```python
from build123d import *

# Parameters (mm, degrees)
SKETCH1_R                   = 12.5
BOSS_EXTRUDE1_DEPTH         = 6.5
CIRPATTERN1_COUNT           = 4
SKETCH5_R                   = 4.5
BOSS_EXTRUDE3_DEPTH         = 6.5
SKETCH7_R                   = 4.1
CUT_EXTRUDE2_DEPTH          = 3
CIRPATTERN3_COUNT           = 2
FILLET2_R                   = 5
M3_TAPPED_HOLE1_D           = 2.5
M3_TAPPED_HOLE1_CSINK_D     = 3.05
M3_TAPPED_HOLE1_CSINK_ANGLE = 90


with BuildPart() as part:
    # Sketch1 → Boss-Extrude1 (new body)
    with BuildSketch(Plane.XY):
        with Locations(Location((0, 0, 0), (0, 0, 180))):
            Circle(SKETCH1_R)
    extrude(amount=BOSS_EXTRUDE1_DEPTH)

    # Sketch4 → CBORE for M3 Hexagon socket head cap screws1 (revolve, cut)
    with BuildSketch(Plane(origin=(-9, 0, 6.5), x_dir=(0, -1, 0), z_dir=(1, 0, 0))):
        Polygon((0, 0), (0, 6.5), (1.6, 6.5), (1.6, 3.4), (3, 3.4), (3, 0.025), (3.025, 0), align=None)
    cbore_for_m3_hexagon_socket_head_cap_scr = revolve(axis=Axis((-9, 0, 12.85), (0, 0, -1)), mode=Mode.SUBTRACT)

    # CirPattern1: CBORE for M3 Hexagon socket head cap screws1 ×4 about axis
    cirpattern1_axis = Axis((0, 0, 0), (0, 0, 1))
    for i in range(1, CIRPATTERN1_COUNT):
        add(cbore_for_m3_hexagon_socket_head_cap_scr.rotate(cirpattern1_axis, i * 360 / CIRPATTERN1_COUNT), mode=Mode.SUBTRACT)

    # Sketch5 → Boss-Extrude3 (add)
    with BuildSketch(Plane.XY.offset(6.5)):
        with Locations((-7.778174593, 7.778174593)):
            Circle(SKETCH5_R)
    boss_extrude3 = extrude(amount=-BOSS_EXTRUDE3_DEPTH)

    # Sketch7 → Cut-Extrude2 (cut)
    with BuildSketch(Plane.XY.offset(6.5)):
        with Locations((-7.778174593, 7.778174593)):
            Circle(SKETCH7_R)
    cut_extrude2 = extrude(amount=-CUT_EXTRUDE2_DEPTH, mode=Mode.SUBTRACT)

    # CirPattern3: Boss-Extrude3, Cut-Extrude2 ×2 about axis
    cirpattern3_axis = Axis((0, 0, 0), (0, 0, 1))
    add([boss_extrude3.rotate(cirpattern3_axis, i * 360 / CIRPATTERN3_COUNT) for i in range(1, CIRPATTERN3_COUNT)])
    add([cut_extrude2.rotate(cirpattern3_axis, i * 360 / CIRPATTERN3_COUNT) for i in range(1, CIRPATTERN3_COUNT)], mode=Mode.SUBTRACT)

    # Fillet2
    fillet2_edges = [part.edges().sort_by_distance(p)[0] for p in [
        (-5.115048509, 11.405537197, 3.25),
        (-11.405537197, 5.115048509, 3.25),
        (5.115048509, -11.405537197, 3.25),
        (11.405537197, -5.115048509, 3.25),
    ]]
    fillet(fillet2_edges, radius=FILLET2_R)

    # M3 Tapped Hole1 (through all)
    with Locations(Plane(origin=(-7.778174593, 7.778174593, 3.5), x_dir=(1, 0, 0), z_dir=(0, 0, 1))):
        with Locations((0, 0), (15.556349186, -15.556349186)):
            CounterSinkHole(M3_TAPPED_HOLE1_D / 2, M3_TAPPED_HOLE1_CSINK_D / 2, counter_sink_angle=M3_TAPPED_HOLE1_CSINK_ANGLE)


solid = part.part
```
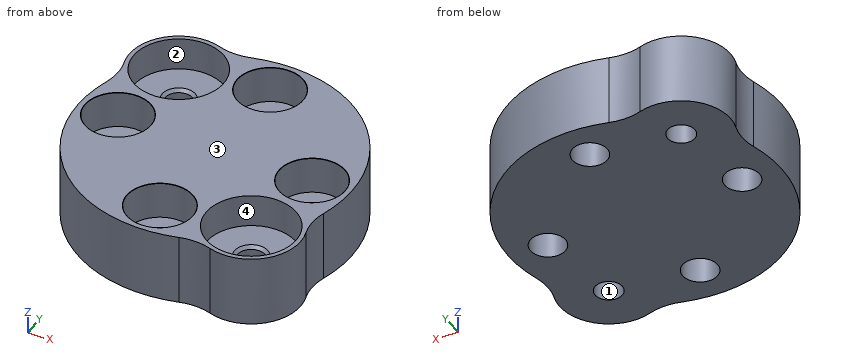
Input: part model. Units: mm. Frame: model coordinates. Face numbers are marked on the shaded views. A direction names the side the tool comes from. Round coordinates to 2 decimals unless told otherwise and drop trailing zeros. Write each loop counter-clockwise with the first axis right and the second up, starting at its lowest first coordinate (ties: lowest second). Pieces come first, ordered by that corner, then holes. Notation, with made-up numbers: (23, -8) -> (73, -8) arc R18 cw to (73, 14) -> close; hole circle Ø7 at (84.5, -12). An arc over 180 degrees is marked (long way). Answer as CSV lines item,"result".
1. Section A-A (x = 0). Return the cut outline in (y, z) (3 decimals).
Geometry says:
outline,"(-12.5, 0) -> (-10.6, 0) -> (-10.6, 3.1) -> (-12, 3.1) -> (-12, 6.475) -> (-12.025, 6.5) -> (-12.5, 6.5) -> close; (-7.4, 0) -> (7.4, 0) -> (7.4, 3.1) -> (6, 3.1) -> (6, 6.475) -> (5.975, 6.5) -> (-5.975, 6.5) -> (-6, 6.475) -> (-6, 3.1) -> (-7.4, 3.1) -> close; (10.6, 0) -> (12.5, 0) -> (12.5, 6.5) -> (12.025, 6.5) -> (12, 6.475) -> (12, 3.1) -> (10.6, 3.1) -> close"
2. Section C-C (z = 4). Give the number of separate pieces and of enclosed holes in the cut face, plus the area to 3 significant figures.
Geometry says:
separate pieces,"1"
enclosed holes,"6"
area,"315 mm^2"
3. Reachability of the marked faces 1 and 2 from +Z, -Z, +X, -X, +Y, -Y: full face, straight path, thin tool, end or side. Return the list, or none.
Geometry says:
face 1,"+Z, -Z"
face 2,"+Z"
4. Ray query, L1, parallel to X at y = 0, z = 2.2; L2, parallel to X at y = 0, z = 5.25. Return the intervals inside material, ascending. Write a range as [from, to].
Geometry says:
L1,"x = [-12.5, -10.6], [-7.4, 7.4], [10.6, 12.5]"
L2,"x = [-12.5, -12], [-6, 6], [12, 12.5]"
5. Mould query, pull axis X, two halves, no side actions, for the marked faces 3 and 4. Classes: +X half, -X half, draft (parallel to the pull), parting line (faces both ways), or undercut.
Geometry says:
face 3,"draft"
face 4,"undercut"
6. Contact query for flat-ended pins moving along their axis: P1, Ø5, axis at x = 9, y = 0, coming from the +Z side; P2, Ø1.9, axis at x = -9, y = 0, coming from the +Z side; P3, Ø4, axis at x = 7.5, y = -9, coming from the +Z side; P4, Ø1.5, axis at x = -8, z = 4, coming from the +Y side. Output: stop coordinate, or through.
Geometry says:
P1,"stops at z = 3.1"
P2,"passes through"
P3,"stops at z = 3.5"
P4,"stops at y = 12.28"
